from build123d import *

# Parameters (mm, degrees)
F0_W      = 254
F0_H      = 190.5
F1_DEPTH  = 85.725
F3_DEPTH  = 127
F4_R      = 9.525
F5_DEPTH  = 12.7
F6_R      = 6.35
F7_DEPTH  = 85.725
F8_R      = 6.35
F9_R      = 6.35
F10_DEPTH = 82.55
F12_D     = 12.7
F12_DEPTH = 31.75
F12_TIP   = 3.8154649308
F14_D     = 12.7
F14_DEPTH = 31.75
F14_TIP   = 3.8154649308


with BuildPart() as f1:
    # F0 (on Front) → F1 (new body)
    with BuildSketch(Plane.XZ):
        Rectangle(F0_W, F0_H)
    extrude(amount=-F1_DEPTH)

    # F2 (on Right) → F3 (cut, symmetric)
    with BuildSketch(Plane.YZ):
        with BuildLine():
            Line((0, 0), (0, -50.8))
            ThreePointArc((0, -50.8), (50.8, 0), (0, 50.8))
            Line((0, 50.8), (0, 0))
        make_face()
    extrude(amount=F3_DEPTH, both=True, mode=Mode.SUBTRACT)

    # F4 (on face) → F5 (cut)
    with BuildSketch(Plane.XZ):
        with Locations((-73.025, 73.025)):
            Circle(F4_R)
        with Locations((-73.025, -73.025)):
            Circle(F4_R)
        with Locations((101.6, 73.025)):
            Circle(F4_R)
        with Locations((101.6, -73.025)):
            Circle(F4_R)
    extrude(amount=-F5_DEPTH, mode=Mode.SUBTRACT)

    # F6 (on face) → F7 (cut, through all)
    with BuildSketch(Plane.XZ):
        with Locations((-49.2125, 73.025)):
            Circle(F6_R)
        with Locations((77.7875, -73.025)):
            Circle(F6_R)
    extrude(amount=-F7_DEPTH, mode=Mode.SUBTRACT)

    # F8 (on face) + F9 (on face) → F10 (cut)
    with BuildSketch(Plane.XZ.offset(-12.7)):
        with Locations((-73.025, 73.025)):
            Circle(F8_R)
        with Locations((-73.025, -73.025)):
            Circle(F8_R)
    with BuildSketch(Plane.XZ.offset(-12.7)):
        with Locations((101.6, 73.025)):
            Circle(F9_R)
        with Locations((101.6, -73.025)):
            Circle(F9_R)
    extrude(amount=-F10_DEPTH, mode=Mode.SUBTRACT)

    # F12
    with Locations(Plane.XY.offset(95.25)):
        with Locations((-11.1125, 66.675), (36.5125, 66.675)):
            Hole(F12_D / 2, depth=F12_DEPTH)
            with Locations((0, 0, -(F12_DEPTH + F12_TIP / 2))):  # 118° drill point
                Cone(0, F12_D / 2, F12_TIP, mode=Mode.SUBTRACT)

    # F14
    with Locations(Plane.YZ.offset(127)):
        with Locations((66.675, 50.8), (66.675, -50.8)):
            Hole(F14_D / 2, depth=F14_DEPTH)
            with Locations((0, 0, -(F14_DEPTH + F14_TIP / 2))):  # 118° drill point
                Cone(0, F14_D / 2, F14_TIP, mode=Mode.SUBTRACT)


solid = f1.part
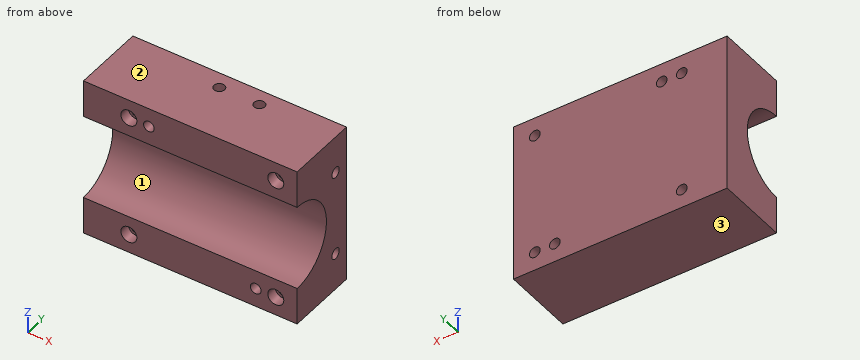
Could you check a few things on this model? Use its own coordinates, in mm. Face numbers are marked on the shaded views. Round coordinates to 2 decimals unless told otherwise and drop trailing zeros. Order: outer loops, then holes, each group sorted by start corner. A loop starts at its lowest first (then second) coordinate and runs counter-clockwise, first axis right, second up. Notation, with made-up numbers: M 59,84.5 L 94,84.5 A19 cw 94,112.5 Z; hole C -12.5,1 d7. An arc over 180 degrees is marked long. One line per item, written item: value.
(1) Imagine slicing it at A-A (y = 15.5). Count the separate pieces of the cut face and the enclosed holes in it, and give its area (3 significant figures).
Ans:
separate pieces: 2
enclosed holes: 6
area: 23,100 mm^2
(2) Imagine slicing it at B-B (x = 59.5). Write out the boundary of the cut face in (y, z) (3 decimals), and give its area (3 significant figures).
Ans:
outline: M 0,-95.25 L 85.725,-95.25 L 85.725,95.25 L 0,95.25 L 0,50.8 A50.8 cw 0,-50.8 Z
area: 12,300 mm^2
(3) If we mould it in two halves opening along Z, with no side actions, what happens to the marked faces 1, 2 and 3? For each: released by +Z, released by -Z, zero draft, split by the parting line, or undercut.
Ans:
face 1: undercut
face 2: released by +Z
face 3: released by -Z
(4) I need wall thicknesses on line 1 along Z through (x, y) = (101, 59); line 2 along Z through (x, y) = (101.6, 2.5); line 3 along Z through (x, y) = (-76, 16). Which ranges of each line are inside material? Lowest first, please. Write a range as from..to.
Ans:
line 1: z = -95.25..-79.35, -66.7..66.7, 79.35..95.25
line 2: z = -95.25..-82.55, -63.5..-50.74, 50.74..63.5, 82.55..95.25
line 3: z = -95.25..-78.63, -67.42..-48.21, 48.21..67.42, 78.63..95.25
(5) Imagine slicing it at C-C (z = 0). Write out the boundary of the cut face in (x, y) (3 decimals).
Ans:
outline: M -127,50.8 L 127,50.8 L 127,85.725 L -127,85.725 Z
(6) I'm going to push flat-ended pins straight in: P1, Ø2, axis at x = -40, z = 23, coming from the -Y side; P2, Ø10, axis at y = 66.675, z = -50.8, coming from the +X side; P3, Ø15, axis at x = -73.025, z = 73.025, coming from the -Y side; P4, Ø10, axis at x = -73.025, z = 73.025, coming from the +Y side. Where does each tip first touch, or does it pass through?
Ans:
P1: stops at y = 44.77
P2: stops at x = 94.44
P3: stops at y = 12.7
P4: passes through
